```python
from build123d import *

# Parameters (mm, degrees)
ESBO_O1_R                = 1
ESBO_O1_R_2              = 0.5
RESSALTO_EXTRUS_O1_DEPTH = 6
ESBO_O3_R                = 3.5
RESSALTO_EXTRUS_O2_DEPTH = 3
ESBO_O4_R                = 3
CORTE_EXTRUS_O1_DEPTH    = 2
CHANFRO1_SIZE            = 1


with BuildPart() as part:
    # Esboço1 → Ressalto-extrusão1 (new body)
    with BuildSketch(Plane.XY):
        Circle(ESBO_O1_R)
        Circle(ESBO_O1_R_2, mode=Mode.SUBTRACT)
    extrude(amount=RESSALTO_EXTRUS_O1_DEPTH)

    # Esboço3 → Ressalto-extrusão2 (add)
    with BuildSketch(Plane.XY.offset(6)):
        Circle(ESBO_O3_R)
    extrude(amount=RESSALTO_EXTRUS_O2_DEPTH)

    # Esboço4 → Corte-extrusão1 (cut)
    with BuildSketch(Plane.XY.offset(9)):
        Circle(ESBO_O4_R)
    extrude(amount=-CORTE_EXTRUS_O1_DEPTH, mode=Mode.SUBTRACT)

    # Chanfro1
    # the kernel refuses this chamfer: 1 mm, written as the material it takes off along each edge
    with BuildSketch(Plane(origin=(0, 0, 9), x_dir=(1, 0, 0), z_dir=(0, -1, 0))) as chanfro1_piece_1:
        Polygon((3.5, -CHANFRO1_SIZE), (3.5 - CHANFRO1_SIZE, 0), (3.5, 0), align=None)
    revolve(axis=Axis((0, 0, 9), (0, 0, 1)), mode=Mode.SUBTRACT)
    with BuildSketch(Plane(origin=(0, 0, 6), x_dir=(1, 0, 0), z_dir=(0, -1, 0))) as chanfro1_piece_2:
        Polygon((3.5, CHANFRO1_SIZE), (3.5 - CHANFRO1_SIZE, 0), (3.5, 0), align=None)
    revolve(axis=Axis((0, 0, 6), (0, 0, 1)), mode=Mode.SUBTRACT)


solid = part.part
```
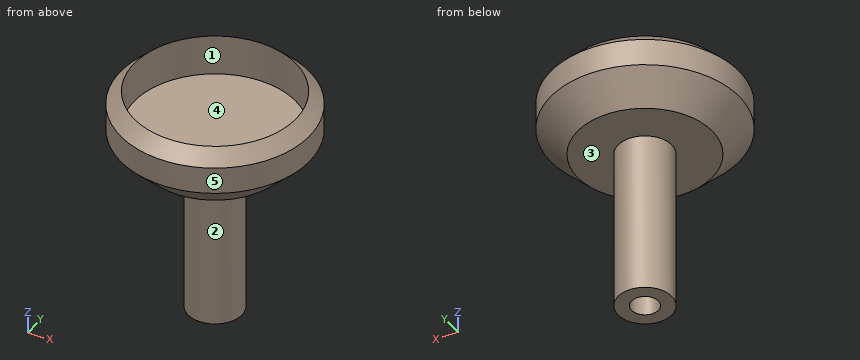
Could you check a few things on this model? Use its own coordinates, in mm. Face numbers are marked on the shaded views. A direction names the side the tool comes from. Round coordinates to 2 decimals unless told otherwise and drop trailing zeros. Write each loop counter-clockwise with the first axis right and the second up, starting at its lowest first coordinate (ties: lowest second). Pieces come first, ordered by that corner, then holes.
(1) Thinking about a two-plate mould opening in X: for the marked faces 3, 4 and 5, which applies, +X half, -X half, draft (parallel to the pull), parting line (faces both ways), or undercut?
Findings below:
face 3: draft
face 4: undercut
face 5: parting line
(2) If I drill on probe 1 along Y at (x, z) = (0, 2.6); probe 2 along Y at (x, z) = (0, 7.8); probe 3 along Z at (x, y) = (-0.25, 1), over which ranges is the centre line in solid material (lowest first)?
Findings below:
probe 1: y = -1 to -0.5, 0.5 to 1
probe 2: y = -3.5 to -3, 3 to 3.5
probe 3: z = 6 to 7
(3) Suppose I cut it at A-A on x = 0. Write out the boundary of the cut face in (y, z).
Findings below:
outline: (-3.5, 7) - (-2.5, 6) - (-1, 6) - (-1, 0) - (-0.5, 0) - (-0.5, 6) - (0.5, 6) - (0.5, 0) - (1, 0) - (1, 6) - (2.5, 6) - (3.5, 7) - (3.5, 8) - (3, 8.5) - (3, 7) - (-3, 7) - (-3, 8.5) - (-3.5, 8) - close
(4) Suppose I cut it at D-D on z = 6.75. Write out the boundary of the cut face in (x, y).
Findings below:
outline: circle Ø6.5 at (0, 0)
(5) Suppose I cut it at C-C on z = 1. Write out the boundary of the cut face in (x, y), and give its area (3 significant figures).
Findings below:
outline: circle Ø2 at (0, 0); hole circle Ø1 at (0, 0)
area: 2.36 mm2
(6) For pin 1 (2 mm diameter, centred on x = 2.5, y = 0.5, fed in from -Z); pin 2 (1.5 mm diameter, centred on y = -2, z = 2.5, fed in from -X); pin 3 (1.5 mm diameter, centred on y = 1, z = 5.5, fed in from -X), each with a flat end and sliding along its axis, tell me the tip position at first contact or that it passes through.
Findings below:
pin 1: stops at z = 6
pin 2: passes through
pin 3: stops at x = -2.6
(7) Which directions (+Z, -Z, +X, -X, +Y, -Y) give clear straight access to the entire face, cutting with the end or side of a thin tool? Please do the marked faces 1 and 2.
Findings below:
face 1: +Z
face 2: -Z
